Verification items for this drawing (mm, ordinates from the low corner). A direction names the side the tool comes from. Coordinates: 2 decimals unless noted, no trailing zeros. Write each loop counter-clockwise with the first axis right and the second up, starting at its lowest first coordinate (ties: lowest second). Pieces come first, ordered by that corner, then holes. Notation, with made-up numbers: M 38.25,15 L 70.25,15 A10 ccw 70.25,30 Z; hole C 89.5,-31.75 d9. An arc over 180 degrees is marked long. Answer as CSV lines item,"result". Start each with the question number.
1) Access from +Z, -Z, +X, -X, +Y, -Y to the whole of each face (thin tool, end or side, straight path). Record for the marked faces 1 and 2.
2) Go/stop test with flat-tipped pins: pin 1 Ø6 at (y, z) = (43, 41) entering from -X; pin 2 Ø4 at (x, z) = (7.5, 26) entering from +Y; pin 3 Ø22 at (x, y) = (32.5, 79) entering from -Z. Record where each tip stops, or that it passes through.
3) Section check C-C (x = 28). Record the cut outline in (y, z), and give its area (3 significant figures).
4) Section check D-D (y = 25). Record the cut outline in (x, z), and give its area (3 significant figures).
5) Material ranges on L1, parallel to Z at x = 10, y = 3; L2, parallel to X at y = 8, z = 10; L3, parallel to X at y = 7, z = 27, recorded low to high. Write a range as [from, to].
6) Section check A-A (z = 10.16). Record the cut outline in (x, y) (3 decimals), and give its area (3 significant figures).
7) Section check B-B (x = 10.16). Record the cut outline in (y, z) (3 decimals), and give its area (3 significant figures).
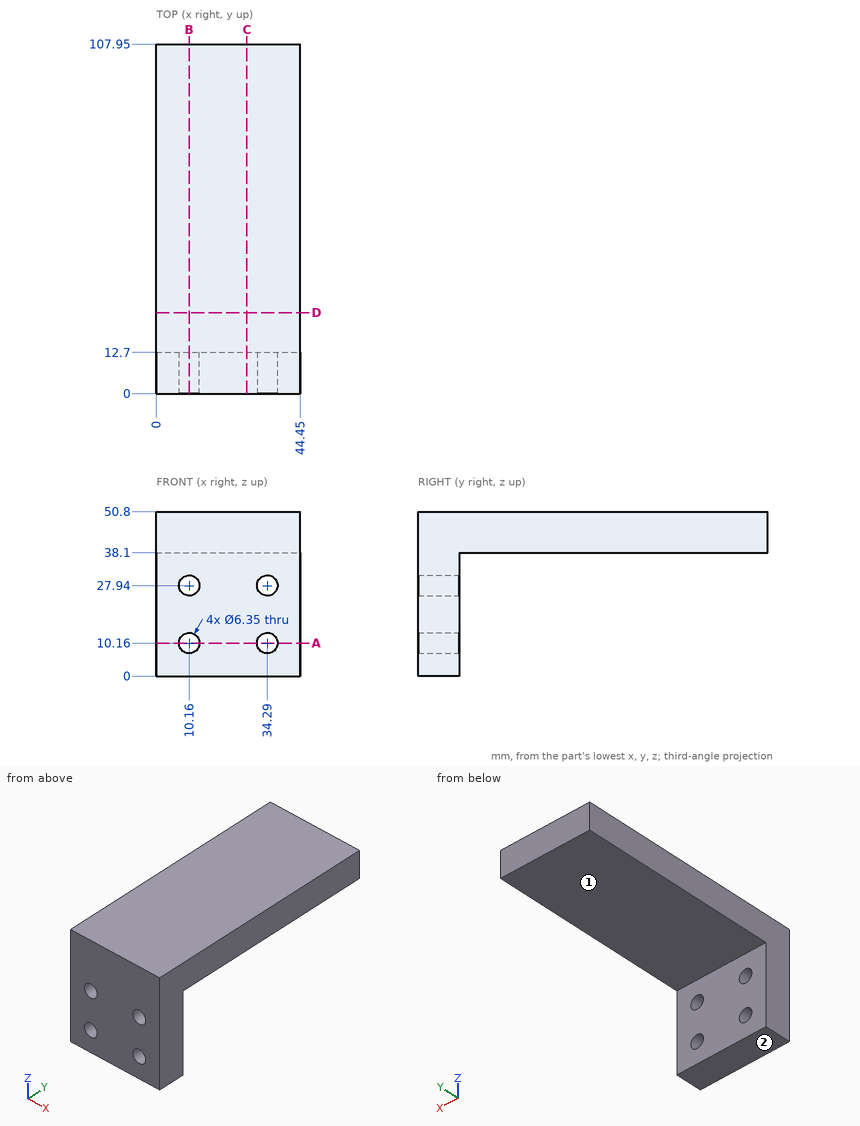
Results found:
1,face 1,"-Z, +X, -X, +Y"
1,face 2,"-Z, +X, -X, +Y, -Y"
2,pin 1,"stops at x = 0"
2,pin 2,"stops at y = 12.7"
2,pin 3,"stops at z = 38.1"
3,outline,"M 0,0 L 12.7,0 L 12.7,38.1 L 107.95,38.1 L 107.95,50.8 L 0,50.8 Z"
3,area,"1,850 mm2"
4,outline,"M 0,38.1 L 44.45,38.1 L 44.45,50.8 L 0,50.8 Z"
4,area,"565 mm2"
5,L1,"z = [0, 6.99], [13.33, 24.77], [31.11, 50.8]"
5,L2,"x = [0, 6.99], [13.33, 31.12], [37.46, 44.45]"
5,L3,"x = [0, 7.13], [13.19, 31.26], [37.32, 44.45]"
6,outline,"M 0,0 L 6.985,0 L 6.985,12.7 L 0,12.7 Z; M 13.335,0 L 31.115,0 L 31.115,12.7 L 13.335,12.7 Z; M 37.465,0 L 44.45,0 L 44.45,12.7 L 37.465,12.7 Z"
6,area,"403 mm2"
7,outline,"M 0,0 L 12.7,0 L 12.7,6.985 L 0,6.985 Z; M 0,13.335 L 12.7,13.335 L 12.7,24.765 L 0,24.765 Z; M 0,31.115 L 12.7,31.115 L 12.7,38.1 L 107.95,38.1 L 107.95,50.8 L 0,50.8 Z"
7,area,"1,690 mm2"
